```python
from build123d import *

# Parameters (mm, degrees)
F0_R     = 11.1125
F1_DEPTH = 41.9481
F3_DEPTH = 9.525
F5_D     = 7.9375
F5_DEPTH = 34.7472
F5_TIP   = 2.3846655818
F6_R     = 1.905


with BuildPart() as f1:
    # F0 (on Right) → F1 (new body)
    with BuildSketch(Plane.YZ):
        Circle(F0_R)
    extrude(amount=-F1_DEPTH)

    # F2 (on Right) → F3 (cut)
    with BuildSketch(Plane.YZ):
        Polygon((4.7879, -2.7642953539), (4.7879, 2.7642953539), (0, 5.5285907077), (-4.7879, 2.7642953539), (-4.7879, -2.7642953539), (0, -5.5285907077), align=None)
    extrude(amount=-F3_DEPTH, mode=Mode.SUBTRACT)

    # F5
    with Locations(Plane(origin=(-41.9481, 0, 0), x_dir=(0, -1, 0), z_dir=(-1, 0, 0))):
        with Locations((0, 0)):
            Hole(F5_D / 2, depth=F5_DEPTH)
            with Locations((0, 0, -(F5_DEPTH + F5_TIP / 2))):  # 118° drill point
                Cone(0, F5_D / 2, F5_TIP, mode=Mode.SUBTRACT)

    # F6 (on Front) → F7 (revolve, cut)
    with BuildSketch(Plane.XZ):
        with Locations((-29.2481, 11.1125)):
            Circle(F6_R)
    revolve(axis=Axis((-32.1425274014, 0, 0), (-1, 0, 0)), mode=Mode.SUBTRACT)


solid = f1.part
```
Check sheet for the modelled part. Datum: model origin and axes. Units: mm. A direction names the side the tool comes from. Round coordinates to 2 decimals unless told otherwise and drop trailing zeros. Loops run counter-clockwise (first coordinate to the right, second up) from the corner with the lowest first, then second, coordinate; pieces in that order, holes last. Notation, with made-up numbers: (9, -39) - (68, -39) arc R22 ccw to (68, -2) - close; hole circle Ø10 at (10, 80). An arc over 180 degrees is marked (long way). Answer as a JSON object with one key per item and string values. Group by question number.
Q1. Sectioned sample at A-A, the plane z = 0. Enter the section's corners in (x, y) (1 decimal), plus the area to 3 significant figures.
Q2. Mould release check, pull along Z, two halves, no side actions. Record for faces 1 (the face through (-36.48, 10.6, 3.34)), 2 (the face through (-5, 4.788, 0)), 3 (the face through (-41.948, 0, -5)), 4 (the face through (-4.696, -2.36, 4.166)): released by +Z, released by -Z, zero draft, split by the parting line, or undercut.
Q3. Sectioned sample at B-B, the plane x = -4. Enter the section's corners in (y, z) (1 decimal), plus the area to 3 significant figures.
Q4. Set-up check for faces 5 (the face through (-13.48, 10.6, 3.34)), 6 (the face through (-4.696, 2.36, -4.166)): record each of +Z, -Z, +X, -X, +Y, -Y from which the full face is reachable in a straight line by a thin tool's end or side.
Q5. Gauge pin test, flat ends, axial feed: P1, Ø5, axis at x = -23.5, y = -5, coming from the +Z side; P2, Ø4, axis at x = -33.5, z = -6, coming from the -Y side; P3, Ø1, axis at x = -8, y = -7.5, coming from the +Z side. Record the tip position at first contact, or that the pin passes through.
Q6. Sectioned sample at C-C, the plane x = -23.5. Enter the section's corners in (y, z) (1 decimal).
Q7. Scan lines: line 1 along Z through (x, y) = (-25, 0); line 2 along X through (y, z) = (4.75, 1.5) (3 decimals); line 3 along Z through (x, y) = (-24.5, -2). Record each from-to range of solid material in increasing order. Write a range as [from, to].
Solution:
{
 "1": {"outline": "(-41.9, -11.1) - (-31.2, -11.1) arc R1.9 cw to (-27.3, -11.1) - (0, -11.1) - (0, -4.8) - (-9.5, -4.8) - (-9.5, -4) - (-41.9, -4) - close; (-41.9, 4) - (-9.5, 4) - (-9.5, 4.8) - (0, 4.8) - (0, 11.1) - (-27.3, 11.1) arc R1.9 cw to (-31.2, 11.1) - (-41.9, 11.1) - close", "area": "572 mm²"},
 "2": {"face 1": "split by the parting line", "face 2": "undercut", "face 3": "zero draft", "face 4": "undercut"},
 "3": {"outline": "circle Ø22.2 at (0, 0); hole (-4.8, -2.8) - (0, -5.5) - (4.8, -2.8) - (4.8, 2.8) - (0, 5.5) - (-4.8, 2.8) - close", "area": "309 mm²"},
 "4": {"face 5": "+X, -X", "face 6": "+X"},
 "5": {"P1": "stops at z = 10.83", "P2": "stops at y = -10.37", "P3": "stops at z = 8.63"},
 "6": {"outline": "circle Ø22.2 at (0, 0); hole circle Ø7.9 at (0, 0)"},
 "7": {"line 1": "z = [-11.11, -3.97], [3.97, 11.11]", "line 2": "x = [-41.948, -9.525]", "line 3": "z = [-10.93, -3.43], [3.43, 10.93]"}
}
